```python
from build123d import *

# Parameters (mm, degrees)
SKETCH_1_W          = 6.32
SKETCH_1_H          = 6.32
SKETCH_1_R          = 0.1861223
EXTRUDE_1_DEPTH     = 165.1
FILLET_1_R          = 1
SKETCH_2_R          = 2.1
CUT_EXTRUDE_1_DEPTH = 165.1


with BuildPart() as part:
    # 草图1 → 凸台-拉伸1 (new body)
    with BuildSketch(Plane(origin=(0, 0, 0), x_dir=(0, 0, -1), z_dir=(1, 0, 0))):
        Rectangle(SKETCH_1_W, SKETCH_1_H)
        Circle(SKETCH_1_R, mode=Mode.SUBTRACT)
    extrude(amount=EXTRUDE_1_DEPTH)

    # 圆角1
    fillet_1_edges = [part.edges().sort_by_distance(p)[0] for p in [
        (82.55, -3.16, -3.16),
        (82.55, -3.16, 3.16),
        (82.55, 3.16, 3.16),
        (82.55, 3.16, -3.16),
    ]]
    fillet(fillet_1_edges, radius=FILLET_1_R)

    # 草图2 → 切除-拉伸1 (cut)
    with BuildSketch(Plane(origin=(0, 0, -3.16), x_dir=(-1, 0, 0), z_dir=(0, 0, -1))):
        with Locations((-161.692066873, -0.018189101)):
            Circle(SKETCH_2_R)
        with Locations((-110.892066873, -0.018189101)):
            Circle(SKETCH_2_R)
    extrude(amount=-CUT_EXTRUDE_1_DEPTH, mode=Mode.SUBTRACT)


solid = part.part
```
Geometry: final body of the model. Coordinates: model frame, mm. Round coordinates to 2 decimals unless told otherwise and drop trailing zeros. Write each loop counter-clockwise with the first axis right and the second up, starting at its lowest first coordinate (ties: lowest second). Pieces come first, ordered by that corner, then holes. Notation, with made-up numbers: (83.5, 85.25) -> (129.5, 85.25) arc R12 ccw to (129.5, 105.25) -> close; hole circle Ø3 at (-33.75, 12.5). An arc over 180 degrees is marked (long way). Use CSV: the item, a comma, the result in double quotes. Start each with the question number.
Q1. Section A-A (x = 141.5). Return loops of the section in (y, z), plus the area to 3 significant figures.
Q2. Line query: L1, parallel to X at y = 0, z = -1.25; L2, parallel to Z at x = 148, y = 0; L3, parallel to X at y = 0.5, z = 2. Output: solid intervals per line, ascending.
Q3. Pull-direction query (Y, two-part tool) for faces 1 (the face through (81, -3.16, 0)), 2 (the face through (81, 0, -3.16)), 3 (the face through (159.69, 0.61, -0.04)); classes: pulls with the +Y half, pulls with the -Y half, needs draft (parallel to the pull), parting line crosses it, or undercut.
Result sheet:
1,outline,"(-3.16, -2.16) arc R1 ccw to (-2.16, -3.16) -> (2.16, -3.16) arc R1 ccw to (3.16, -2.16) -> (3.16, 2.16) arc R1 ccw to (2.16, 3.16) -> (-2.16, 3.16) arc R1 ccw to (-3.16, 2.16) -> close; hole circle Ø0.37 at (0, 0)"
1,area,"39.0 mm²"
2,L1,"0 to 108.79, 112.99 to 159.59, 163.79 to 165.1"
2,L2,"-3.16 to -0.19, 0.19 to 3.16"
2,L3,"0 to 108.86, 112.93 to 159.66, 163.73 to 165.1"
3,face 1,"pulls with the -Y half"
3,face 2,"needs draft"
3,face 3,"undercut"
